Design review of the part built by this model. Coordinates are the model's own, in mm. A direction names the side the tool comes from. Coordinates: 2 decimals unless noted, no trailing zeros. Order: outer loops, then holes, each group sorted by start corner. A loop starts at its lowest first (then second) coordinate and runs counter-clockwise, first axis right, second up. Notation, with made-up numbers: M 67,-11 L 72,-11 A14 cw 72,1 Z; hole C -8,76.5 d5. An arc over 180 degrees is marked long. Answer as a JSON object with one key per item and string values.
from build123d import *

# Parameters (mm, degrees)
SKETCH_6_W          = 18
SKETCH_6_H          = 37.22
SKETCH_6_R          = 4.5
SKETCH_6_R_2        = 2.1
EXTRUDE_2_DEPTH     = 42.1
SKETCH_8_W          = 14.7
SKETCH_8_H          = 37.22
SKETCH_8_W_2        = 13.4
CUT_EXTRUDE_1_DEPTH = 42.1


with BuildPart() as part:
    # 草图6 → 凸台-拉伸2 (new body)
    with BuildSketch(Plane.XY):
        with Locations((424.099665512, 777.503186937)):
            Rectangle(SKETCH_6_W, SKETCH_6_H)
        with Locations((424.099665512, 770.113186937)):
            Circle(SKETCH_6_R, mode=Mode.SUBTRACT)
        with Locations((424.099665512, 787.113186937)):
            Circle(SKETCH_6_R, mode=Mode.SUBTRACT)
        with BuildLine():
            ThreePointArc((433.099665512, 753.358417872), (431.714665512, 751.193186937), (433.099665512, 749.027956002))
            Line((433.099665512, 749.027956002), (433.099665512, 747.193186937))
            Line((433.099665512, 747.193186937), (415.099665512, 747.193186937))
            Line((415.099665512, 747.193186937), (415.099665512, 749.027956002))
            ThreePointArc((415.099665512, 749.027956002), (416.484665512, 751.193186937), (415.099665512, 753.358417872))
            Line((415.099665512, 753.358417872), (415.099665512, 758.893186937))
            Line((415.099665512, 758.893186937), (433.099665512, 758.893186937))
            Line((433.099665512, 758.893186937), (433.099665512, 753.358417872))
        make_face()
        with Locations((428.599665512, 754.093186937)):
            Circle(SKETCH_6_R_2, mode=Mode.SUBTRACT)
        with Locations((419.599665512, 754.093186937)):
            Circle(SKETCH_6_R_2, mode=Mode.SUBTRACT)
    extrude(amount=EXTRUDE_2_DEPTH)

    # 草图8 → 切除-拉伸1 (cut)
    with BuildSketch(Plane(origin=(433.099665512, 0, 0), x_dir=(0, 0, -1), z_dir=(1, 0, 0))):
        with Locations((-34.75, 777.503186937)):
            Rectangle(SKETCH_8_W, SKETCH_8_H)
        with Locations((-6.7, 777.503186937)):
            Rectangle(SKETCH_8_W_2, SKETCH_8_H)
    extrude(amount=-CUT_EXTRUDE_1_DEPTH, mode=Mode.SUBTRACT)


solid = part.part
1) Add section C-C (z = 20). State the section outline as (x, y) points (3 decimals), and give its area (3 significant figures).
Taken from the geometry:
{"outline": "M 415.1,747.193 L 433.1,747.193 L 433.1,749.028 A2.385 cw 433.1,753.358 L 433.1,796.113 L 415.1,796.113 L 415.1,753.358 A2.385 cw 415.1,749.028 Z; hole C 419.6,754.093 d4.2; hole C 424.1,770.113 d9; hole C 424.1,787.113 d9; hole C 428.6,754.093 d4.2", "area": "717 mm2"}
2) Add section B-B (z = 35.5). State the section outline as (x, y) points (3 decimals), and give its area (3 significant figures).
Taken from the geometry:
{"outline": "M 415.1,747.193 L 433.1,747.193 L 433.1,749.028 A2.385 cw 433.1,753.358 L 433.1,758.893 L 415.1,758.893 L 415.1,753.358 A2.385 cw 415.1,749.028 Z; hole C 419.6,754.093 d4.2; hole C 428.6,754.093 d4.2", "area": "174 mm2"}
3) Mouldability with a two-part tool opening along Y and no side actions: class faces 4 (the flat face through (424, 753, 0)), 5 (the cylindrical face through (431.715, 751.231, 20.755)), 6 (the flat face through (424, 796.113, 20)) as released by +Y, released by -Y, zero draft, split by the parting line, or undercut.
Taken from the geometry:
{"face 4": "zero draft", "face 5": "undercut", "face 6": "released by +Y"}
4) To check wall thickness, follow L1, parallel to Z at x = 430.75, y = 775.5; L2, parallel to Y at x = 431, z = 34.5; L3, parallel to Y at x = 428, z = 8.5. State the ranges of each line that lie inside material, in increasing order.
Taken from the geometry:
{"L1": "z = 13.4 to 27.4", "L2": "y = 747.19 to 758.89", "L3": "y = 747.19 to 752.08, 756.11 to 758.89"}
5) Add section D-D (x = 428). State the section outline as (y, z) points.
Taken from the geometry:
{"outline": "M 747.19,0 L 752.08,0 L 752.08,42.1 L 747.19,42.1 Z; M 756.11,0 L 758.89,0 L 758.89,13.4 L 767.87,13.4 L 767.87,27.4 L 758.89,27.4 L 758.89,42.1 L 756.11,42.1 Z; M 772.36,13.4 L 784.87,13.4 L 784.87,27.4 L 772.36,27.4 Z; M 789.36,13.4 L 796.11,13.4 L 796.11,27.4 L 789.36,27.4 Z"}
6) Add section A-A (x = 425). State the section outline as (y, z) points, and give its area (3 significant figures).
Taken from the geometry:
{"outline": "M 747.19,0 L 758.89,0 L 758.89,13.4 L 765.7,13.4 L 765.7,27.4 L 758.89,27.4 L 758.89,42.1 L 747.19,42.1 Z; M 774.52,13.4 L 782.7,13.4 L 782.7,27.4 L 774.52,27.4 Z; M 791.52,13.4 L 796.11,13.4 L 796.11,27.4 L 791.52,27.4 Z", "area": "767 mm2"}
7) Tool access review of faces 1 (the flat face through (424, 758.893, 7)), 2 (the flat face through (415.1, 770, 21)), 3 (the flat face through (424, 758.893, 35)): name each direction out of +Z, -Z, +X, -X, +Y, -Y from which nothing blocks a thin tool from reaching the whole face with its end or side.
Taken from the geometry:
{"face 1": "-Z, +X, -X, +Y", "face 2": "+Z, -Z, -X, +Y, -Y", "face 3": "+Z, +X, -X, +Y"}
8) Insertion check: pin 1 Ø5 at (x, y) = (422.5, 766.5) entering from +Z; pin 2 Ø5 at (x, z) = (420.5, 34.5) entering from +Y; pin 3 Ø6.5 at (x, y) = (428.6, 754.09) entering from +Z. Each pin has a flat end and moves straight along its axis. Give the tip position at first contact, or say it passes through.
Taken from the geometry:
{"pin 1": "stops at z = 27.4", "pin 2": "stops at y = 758.89", "pin 3": "stops at z = 42.1"}
